Geometry check sheet. Reference: the model listing, model coordinates, mm. Face numbers are marked on the shaded views. A direction names the side the tool comes from. Give positions to 0.01 mm unless a question says otherwise; leave off trailing zeros. Write each loop counter-clockwise with the first axis right and the second up, starting at its lowest first coordinate (ties: lowest second). Pieces come first, ordered by that corner, then holes. Notation, with made-up numbers: M 22,-35 L 77,-35 A27 cw 77,-16 Z; hole C 2,64 d2. An arc over 180 degrees is marked long. One line per item, written item: value. Start each with the question number.
1. Cross-section at A-A on y = 1. Record the cut outline in (x, z) (3 decimals), then the cut area to 3 significant figures.
2. Cross-section at C-C on y = 7. Record the cut outline in (x, z).
3. Cross-section at D-D on z = 22. Record the cut outline in (x, y) (3 decimals).
4. Scan lines: line 1 (X direction, y = -5, z = 10); line 2 (Y direction, x = 4, z = 21) (3 decimals); line 3 (Z direction, x = -7.25, y = -4.25). Record each from-to range of solid material in increasing order.
5. Cross-section at B-B on x = -0.5. Record the cut outline in (y, z) (1 decimal), then the cut area to 3 significant figures.
6. Gauge pin test, flat ends, axial feed: pin 1 (3 mm diameter, centred on y = -0.5, z = 0, fed in from +X); pin 2 (2.5 mm diameter, centred on x = 0, y = -6, fed in from +Z); pin 3 (2.5 mm diameter, centred on x = 0, z = 21.46, fed in from +Y); pin 4 (2 mm diameter, centred on x = 3, y = 1.5, fed in from -Z). Record the tip position at first contact, or that the pin passes through.
7. Tool access check on the marked faces 4, 5 and 6. Record the directions out of +Z, -Z, +X, -X, +Y, -Y that give a thin tool (end or side, any length) a straight path to the whole face; none if there is none.
8. Release check for a two-part mould opening along Z. For the marked faces 1, 2 and 3 record: pulls with the +Z half, pulls with the -Z half, needs draft (parallel to the pull), parting line crosses it, or undercut.
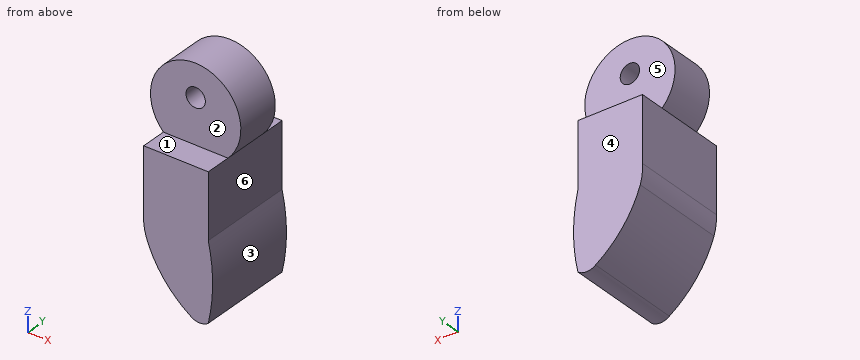
from build123d import *

# Parameters (mm, degrees)
SKETCH1_W                = 12.7
SKETCH1_H                = 19.05
BOSS_EXTRUDE1_DEPTH      = 12.7
BOSS_EXTRUDE3_DEPTH      = 4.445
BOSS_EXTRUDE3_DEPTH_BACK = 14.605
BOSS_EXTRUDE5_DEPTH      = 4.445
SKETCH9_R                = 1.905
CUT_EXTRUDE1_DEPTH       = 8.89


with BuildPart() as part:
    # Sketch1 → Boss-Extrude1 (new body)
    with BuildSketch(Plane.XY):
        Rectangle(SKETCH1_W, SKETCH1_H)
    extrude(amount=BOSS_EXTRUDE1_DEPTH)

    # Sketch5 → Boss-Extrude3 (add, two sides)
    with BuildSketch(Plane(origin=(0, 5.08, 0), x_dir=(1, 0, 0), z_dir=(0, 1, 0))) as boss_extrude3_sk:
        with BuildLine():
            Line((-6.35, 0), (6.35, 0))
            ThreePointArc((6.35, 0), (7.206801568, 7.62), (6.35, 15.24))
            ThreePointArc((6.35, 15.24), (4.615153625, 15.830989255), (2.88030725, 15.24))
            ThreePointArc((2.88030725, 15.24), (-2.482813439, 10.254375056), (-5.912749562, 3.784826555))
            ThreePointArc((-5.912749562, 3.784826555), (-6.305841352, 1.912568913), (-6.35, 0))
        make_face()
    extrude(amount=BOSS_EXTRUDE3_DEPTH)
    extrude(boss_extrude3_sk.sketch, amount=-BOSS_EXTRUDE3_DEPTH_BACK)

    # Sketch8 → Boss-Extrude5 (add, symmetric)
    with BuildSketch(Plane(origin=(0, 0, 0), x_dir=(1, 0, 0), z_dir=(0, 1, 0))):
        with BuildLine():
            Line((-6.35, -12.7), (6.35, -12.7))
            ThreePointArc((6.35, -12.7), (0, -27.811703947), (-6.35, -12.7))
        make_face()
    extrude(amount=BOSS_EXTRUDE5_DEPTH, both=True)

    # Sketch9 → Cut-Extrude1 (cut)
    with BuildSketch(Plane(origin=(0, 4.445, 0), x_dir=(1, 0, 0), z_dir=(0, 1, 0))):
        with Locations(Location((0, -21.461703947, 0), (0, 0, 270))):  # turned: the seam where the file's is
            Circle(SKETCH9_R)
    extrude(amount=-CUT_EXTRUDE1_DEPTH, mode=Mode.SUBTRACT)


solid = part.part
Report:
1. outline: M -6.35,0 A10.419 ccw -5.913,-3.785 A22.002 ccw 2.88,-15.24 A2.842 ccw 6.35,-15.24 A34.313 ccw 6.35,0 L 6.35,12.7 A8.89 ccw long -6.35,12.7 Z; hole C 0,21.462 d3.81
1. area: 535 mm^2
2. outline: M -6.35,0 A10.42 ccw -5.91,-3.78 A22 ccw 2.88,-15.24 A2.84 ccw 6.35,-15.24 A34.31 ccw 6.35,0 L 6.35,12.7 L -6.35,12.7 Z
3. outline: M -8.34,-4.445 L -1.827,-4.445 L -1.827,4.445 L -8.34,4.445 Z; M 1.827,-4.445 L 8.34,-4.445 L 8.34,4.445 L 1.827,4.445 Z
4. line 1: x = -6.35 to 6.35
4. line 2: y = -4.445 to 4.445
4. line 3: z = 13.78 to 24.07
5. outline: M -9.5,-12.5 L 9.5,-12.5 L 9.5,12.7 L 4.4,12.7 L 4.4,19.6 L -4.4,19.6 L -4.4,12.7 L -9.5,12.7 Z; M -4.4,23.3 L 4.4,23.3 L 4.4,27.8 L -4.4,27.8 Z
5. area: 582 mm^2
6. pin 1: stops at x = 6.66
6. pin 2: stops at z = 12.7
6. pin 3: passes through
6. pin 4: stops at z = -15.76
7. face 4: +Z, -Z, +X, -X, +Y
7. face 5: +Z, +X, -X, +Y
7. face 6: +X, +Y, -Y
8. face 1: pulls with the +Z half
8. face 2: needs draft
8. face 3: undercut
